from build123d import *

# Parameters (mm, degrees)
F0_R     = 30
F0_W     = 8
F0_H     = 8
F1_DEPTH = 10


with BuildPart() as f1:
    # F0 (on Front) → F1 (new body)
    with BuildSketch(Plane.XZ):
        Circle(F0_R)
        with BuildLine():
            Line((-6, -6), (-6, -24.269322))
            ThreePointArc((-6, -24.269322), (-17.67767, -17.67767), (-24.269322, -6))
            Line((-24.269322, -6), (-6, -6))
        make_face(mode=Mode.SUBTRACT)
        with BuildLine():
            Line((6, -6), (24.269322, -6))
            ThreePointArc((24.269322, -6), (17.67767, -17.67767), (6, -24.269322))
            Line((6, -24.269322), (6, -6))
        make_face(mode=Mode.SUBTRACT)
        with BuildLine():
            Line((-6, 24.269322), (-6, 6))
            Line((-6, 6), (-24.269322, 6))
            ThreePointArc((-24.269322, 6), (-17.67767, 17.67767), (-6, 24.269322))
        make_face(mode=Mode.SUBTRACT)
        Rectangle(F0_W, F0_H, mode=Mode.SUBTRACT)
        with BuildLine():
            ThreePointArc((6, 24.269322), (17.67767, 17.67767), (24.269322, 6))
            Line((24.269322, 6), (6, 6))
            Line((6, 6), (6, 24.269322))
        make_face(mode=Mode.SUBTRACT)
    extrude(amount=F1_DEPTH)


solid = f1.part
The listing builds one solid part. Answer for the finished solid, in the listing's coordinates (mm). Coordinates: 2 decimals unless noted, no trailing zeros. Order: outer loops, then holes, each group sorted by start corner. A loop starts at its lowest first (then second) coordinate and runs counter-clockwise, first axis right, second up.
Q1. A cutting plane is placed at A-A, the plane x = 0. Write down the section's boundary in (y, z), and give its area (3 significant figures).
Q2. A cutting plane is placed at B-B, the plane z = 0. Write down the section's boundary in (x, y).
Q3. Consider line 1 (Z direction, x = -0.5, y = -3.25); line 2 (Z direction, x = -12.5, y = -8.25); line 3 (X direction, y = -4.5, z = -20). Determine where each line is inside the solid, lowest interval first.
Q4. A cutting plane is placed at D-D, the plane z = -13. Write down the section's boundary in (x, y).
Q5. A cutting plane is placed at C-C, the plane y = -5. Write down the section's boundary in (x, z), and give its area (3 significant figures).
Q6. For a pull along Z with two mould halves and no side action, classify faces 1 (the face through (6, -10, 0)), 2 (the face through (-17.812, -4.93, 17.543)), 3 (the face through (-29.97, -4.93, 1.32)) as pulls with the +Z half, pulls with the -Z half, needs draft (parallel to the pull), parting line crosses it, or undercut.
Q7. Given P1, Ø5, axis at y = -4, z = -12, coming from the +X side; P2, Ø4, axis at x = 14.5, y = -1.5, coming from the +Z side; P3, Ø2.5, axis at x = 1, y = -4, coming from the +Z side; P4, Ø1, axis at x = 7.5, z = 17, coming from the +Y side, each flat-ended and moving along its own axis, determine where each tip first touches the part or whether it passes through.
Answers follow:
1. outline: (-10, -30) - (0, -30) - (0, -4) - (-10, -4) - close; (-10, 4) - (0, 4) - (0, 30) - (-10, 30) - close
1. area: 520 mm2
2. outline: (-30, -10) - (-4, -10) - (-4, 0) - (-30, 0) - close; (4, -10) - (30, -10) - (30, 0) - (4, 0) - close
3. line 1: z = -30 to -4, 4 to 30
3. line 2: z = -27.27 to -21.65, -6 to 6, 21.65 to 27.27
3. line 3: x = -22.36 to -15, -6 to 6, 15 to 22.36
4. outline: (-27.04, -10) - (-21.35, -10) - (-21.35, 0) - (-27.04, 0) - close; (-6, -10) - (6, -10) - (6, 0) - (-6, 0) - close; (21.35, -10) - (27.04, -10) - (27.04, 0) - (21.35, 0) - close
5. outline: circle Ø60 at (0, 0); hole (-24.27, -6) arc R25 ccw to (-6, -24.27) - (-6, -6) - close; hole (-24.27, 6) - (-6, 6) - (-6, 24.27) arc R25 ccw to start; hole (-4, -4) - (4, -4) - (4, 4) - (-4, 4) - close; hole (6, -24.27) arc R25 ccw to (24.27, -6) - (6, -6) - close; hole (6, 6) - (24.27, 6) arc R25 ccw to (6, 24.27) - close
5. area: 1,840 mm2
6. face 1: needs draft
6. face 2: undercut
6. face 3: parting line crosses it
7. P1: stops at x = 28.46
7. P2: stops at z = 27.27
7. P3: stops at z = 30
7. P4: passes through
